The model under review builds one solid part; all positions refer to its coordinate system, in mm. Coordinates: 2 decimals unless noted, no trailing zeros. Loops run counter-clockwise (first coordinate to the right, second up) from the corner with the lowest first, then second, coordinate; pieces in that order, holes last. Notation, with made-up numbers: M 17,17.5 L 69,17.5 A12 cw 69,22.5 Z; hole C 22.5,54 d11. An arc over 180 degrees is marked long. Write item = value, one per line. Start each with the question number.
Q1. Wall thickness on probe 1 along Z at (x, y) = (93.5, 1.75); probe 2 along Z at (x, y) = (35.5, -0.5); probe 3 along Y at (x, z) = (32.5, 7): over which ranges is each line inside the solid? List them lowest first.
Q2. We need section A-A on y = 0. Give the boundary of the cut face in (x, z) (3 decimals).
Q3. We need section B-B on z = 0. Count the separate pieces of the cut face and the enclosed holes in it, and give its area (3 significant figures).
Q4. Clearance check with a flat-ended pin moving along its axis: pin 1 Ø6 at (x, z) = (72.5, 3.5) entering from -Y. State where the tip first meets the part, or that it passes through.
from build123d import *

# Parameters (mm, degrees)
CROQUIS2_W                = 25.4
CROQUIS2_H                = 6.35
SALIENTE_EXTRUIR1_DEPTH   = 127
TALADRO1_D                = 12.7
CHAFL_N1_SIZE             = 1.5875
MATRIZL1_COUNT            = 6
MATRIZL1_PITCH            = 19.05
CHAFL_N1_OF_MATRIZL1_SIZE = 1.5875


with BuildPart() as part:
    # Croquis2 → Saliente-Extruir1 (new body)
    with BuildSketch(Plane(origin=(0, 0, 0), x_dir=(0, 0, -1), z_dir=(1, 0, 0))):
        Rectangle(CROQUIS2_W, CROQUIS2_H)
    extrude(amount=SALIENTE_EXTRUIR1_DEPTH)

    # Taladro1 (through all)
    with Locations(Plane(origin=(0, 3.175, 0), x_dir=(1, 0, 0), z_dir=(0, 1, 0))):
        with Locations((15.875, 0)):
            taladro1 = Hole(TALADRO1_D / 2)

    # Chaflán1
    chafl_n1_edges = [part.edges().sort_by_distance(p)[0] for p in [
        (22.225, 3.175, 0),
        (22.225, -3.175, 0),
    ]]
    chamfer(chafl_n1_edges, length=CHAFL_N1_SIZE)

    # MatrizL1: Taladro1 ×6
    with Locations(*[(i * MATRIZL1_PITCH, 0, 0) for i in range(1, MATRIZL1_COUNT)]):
        add(taladro1, mode=Mode.SUBTRACT)

    # Chaflán1 of MatrizL1
    chafl_n1_of_matrizl1_edges = [part.edges().sort_by_distance(p)[0] for p in [
        (41.275, 3.175, 0),
        (41.275, -3.175, 0),
        (60.325, 3.175, 0),
        (60.325, -3.175, 0),
        (79.375, 3.175, 0),
        (79.375, -3.175, 0),
        (98.425, 3.175, 0),
        (98.425, -3.175, 0),
        (117.475, 3.175, 0),
        (117.475, -3.175, 0),
    ]]
    chamfer(chafl_n1_of_matrizl1_edges, length=CHAFL_N1_OF_MATRIZL1_SIZE)


solid = part.part
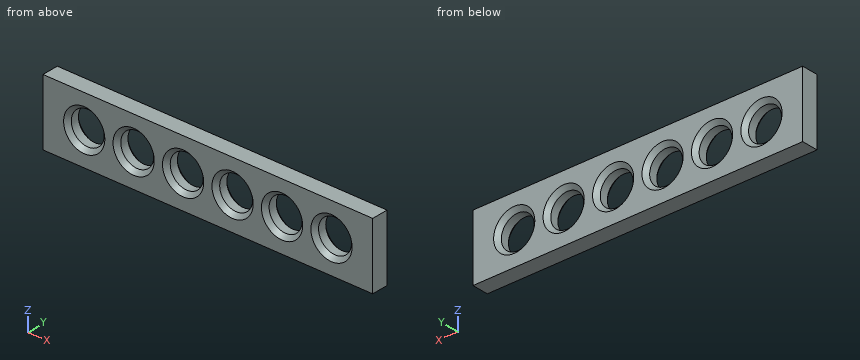
Returned:
q1.probe_1 = -12.7 to -6.35, 6.35 to 12.7
q1.probe_2 = -12.7 to -6.32, 6.32 to 12.7
q1.probe_3 = -2.65 to 2.65
q2.outline = M 0,-12.7 L 127,-12.7 L 127,12.7 L 0,12.7 Z; hole C 15.875,0 d12.7; hole C 34.925,0 d12.7; hole C 53.975,0 d12.7; hole C 73.025,0 d12.7; hole C 92.075,0 d12.7; hole C 111.125,0 d12.7
q3.separate_pieces = 7
q3.enclosed_holes = 0
q3.area = 292 mm^2
q4.pin_1 = -1.78
